from build123d import *

# Parameters (mm, degrees)
SKETCH1_W                       = 15
SKETCH1_H                       = 7.5
SKETCH1_W_2                     = 20
SKETCH1_H_2                     = 27.5
BOSS_EXTRUDE1_DEPTH             = 7
SKETCH2_W                       = 6
SKETCH2_H                       = 7.5
BOSS_EXTRUDE2_DEPTH             = 6
SKETCH8_R                       = 6
BOSS_EXTRUDE4_DEPTH             = 1
SKETCH6_R                       = 1
CUT_EXTRUDE1_DEPTH              = 4
SKETCH7_W                       = 4
SKETCH7_H                       = 11
BOSS_EXTRUDE3_DEPTH             = 4
CBORE_FOR_M5_SBHCS2_D           = 5.5
CBORE_FOR_M5_SBHCS2_CBORE_D     = 9
CBORE_FOR_M5_SBHCS2_CBORE_DEPTH = 1
CHAMFER1_SIZE                   = 2


with BuildPart() as part:
    # Sketch1 → Boss-Extrude1 (new body)
    with BuildSketch(Plane(origin=(0, 0, 0), x_dir=(1, 0, 0), z_dir=(0, 1, 0))):
        with Locations((-7.5, 23.75)):
            Rectangle(SKETCH1_W, SKETCH1_H)
        with Locations((10, 13.75)):
            Rectangle(SKETCH1_W_2, SKETCH1_H_2)
    extrude(amount=BOSS_EXTRUDE1_DEPTH)

    # Sketch2 → Boss-Extrude2 (add)
    with BuildSketch(Plane(origin=(0, 7, 0), x_dir=(1, 0, 0), z_dir=(0, 1, 0))):
        with Locations((-12, 23.75)):
            Rectangle(SKETCH2_W, SKETCH2_H)
    extrude(amount=BOSS_EXTRUDE2_DEPTH)

    # Sketch8 → Boss-Extrude4 (add)
    with BuildSketch(Plane(origin=(0, 7, 0), x_dir=(1, 0, 0), z_dir=(0, 1, 0))):
        with Locations((10, 10)):
            Circle(SKETCH8_R)
    extrude(amount=BOSS_EXTRUDE4_DEPTH)

    # Sketch6 → Cut-Extrude1 (cut)
    with BuildSketch(Plane.ZY.offset(15)):
        with Locations((-25.5, 9.75)):
            Circle(SKETCH6_R)
        with Locations((-25.5, 3.25)):
            Circle(SKETCH6_R)
    extrude(amount=-CUT_EXTRUDE1_DEPTH, mode=Mode.SUBTRACT)

    # Sketch7 → Boss-Extrude3 (add)
    with BuildSketch(Plane.XY.offset(-20)):
        with Locations((-2, 1.5)):
            Rectangle(SKETCH7_W, SKETCH7_H)
    extrude(amount=BOSS_EXTRUDE3_DEPTH)

    # CBORE for M5 SBHCS2 (through all)
    with Locations(Plane(origin=(0, 8, 0), x_dir=(1, 0, 0), z_dir=(0, 1, 0))):
        with Locations((10, 10)):
            CounterBoreHole(CBORE_FOR_M5_SBHCS2_D / 2, CBORE_FOR_M5_SBHCS2_CBORE_D / 2, CBORE_FOR_M5_SBHCS2_CBORE_DEPTH)

    # Chamfer1
    chamfer1_edges = [part.edges().sort_by_distance(p)[0] for p in [
        (-4, -4, -18),
    ]]
    chamfer(chamfer1_edges, length=CHAMFER1_SIZE)


solid = part.part
Read the model definition and answer for the solid it produces. Units are mm, in the model's axes. A direction names the side the tool comes from. Give positions to 0.01 mm unless a question says otherwise; leave off trailing zeros. Write each loop counter-clockwise with the first axis right and the second up, starting at its lowest first coordinate (ties: lowest second). Pieces come first, ordered by that corner, then holes. Notation, with made-up numbers: (71, -15.5) - (89, -15.5) arc R30 cw to (89, 9.5) - close; hole circle Ø8 at (50.5, -39.75). An arc over 180 degrees is marked (long way). Use CSV: the item, a comma, the result in double quotes. Start each with the question number.
(1) Find section D-D (y = 9.75). Give the vertices of the cut face in (x, z), plus the area to 3 significant figures.
(2) Consider line 1 along Y through (x, z) = (-12.8, -25.5); line 2 along Z through (x, y) = (10, 2); line 3 along Y through (x, z) = (-11, -24.5). Determine where each line is inside the solid, lowest interval first.
(3) Find section C-C (z = -10). Give the vertices of the cut face in (x, y).
(4) Find section A-A (y = 1.25). Give the vertices of the cut face in (x, z), plus the area to 3 significant figures.
(5) Find section B-B (x = 10). Give the vertices of the cut face in (y, z), plus the area to 3 significant figures.
(6) Determine the mould class of faces 1 (the flat face through (-2, -2, -20)), 2 (the flat face through (10, 7, -7)), 3 (the flat face through (-12, 13, -24)) for opening direction Z: +Z half, -Z half, draft (parallel to the pull), parting line (faces both ways), or undercut.
(7) For faces 4 (the flat face through (0, -2, -18)), 5 (the flat face through (-9, 10, -24)), 6 (the flat face through (0, 3, -8)), 7 (the flat face through (-11, 3, -26)), 8 (the cylindrical face through (14.292, 7.507, -11.352)), determine the directions among +Z, -Z, +X, -X, +Y, -Y from which every point of the face is accessible in a straight line to the end or side of a thin tool.
(8) Given P1, Ø14, axis at x = 5, z = -11, coming from the +Y side; P2, Ø1.2, axis at y = 3.5, z = -17.5, coming from the -X side; P3, Ø2, axis at x = 1.5, z = -24.5, coming from the +Y side, each flat-ended and moving along its own axis, determine where each tip first touches the part or whether it passes through.
Findings below:
1,outline,"(-15, -27.5) - (-9, -27.5) - (-9, -20) - (-15, -20) - (-15, -24.5) - (-11, -24.5) - (-11, -26.5) - (-15, -26.5) - close"
1,area,"37.0 mm2"
2,line 1,"0 to 2.25, 4.25 to 8.75, 10.75 to 13"
2,line 2,"-27.5 to -12.75, -7.25 to 0"
2,line 3,"0 to 13"
3,outline,"(0, 0) - (7.25, 0) - (7.25, 7) - (5.5, 7) - (5.5, 8) - (4, 8) - (4, 7) - (0, 7) - close; (12.75, 0) - (20, 0) - (20, 7) - (16, 7) - (16, 8) - (14.5, 8) - (14.5, 7) - (12.75, 7) - close"
4,outline,"(-15, -27.5) - (20, -27.5) - (20, 0) - (0, 0) - (0, -16) - (-4, -16) - (-4, -20) - (-15, -20) - close; hole circle Ø5.5 at (10, -10)"
4,area,"655 mm2"
5,outline,"(0, -27.5) - (7, -27.5) - (7, -16) - (8, -16) - (8, -14.5) - (7, -14.5) - (7, -12.75) - (0, -12.75) - close; (0, -7.25) - (7, -7.25) - (7, -5.5) - (8, -5.5) - (8, -4) - (7, -4) - (7, 0) - (0, 0) - close"
5,area,"157 mm2"
6,face 1,"-Z half"
6,face 2,"undercut"
6,face 3,"draft"
7,face 4,"+Z, -Z, +X, -Y"
7,face 5,"+Z, -Z, +X, +Y"
7,face 6,"+Z, -X, +Y, -Y"
7,face 7,"-X"
7,face 8,"+Y"
8,P1,"y = 8"
8,P2,"x = -4"
8,P3,"y = 7"
